Verification items for the finished model (mm, model axes). Round coordinates to 2 decimals unless told otherwise and drop trailing zeros. Write each loop counter-clockwise with the first axis right and the second up, starting at its lowest first coordinate (ties: lowest second). Pieces come first, ordered by that corner, then holes. Notation, with made-up numbers: (-8.75, -32) -> (49.25, -32) arc R25 ccw to (49.25, 6) -> close; hole circle Ø7 at (-40, 44). An arc over 180 degrees is marked (long way). Answer as a JSON object with one key per item and string values. Group by question number.
(1) Sectioned sample at B-B on x = 3.6. Count the separate pieces of the cut face and the enclosed holes in it, and give its area (3 significant figures).
(2) Scan lines: L1, parallel to Z at x = 0.3, y = 90.5; L2, parallel to Z at x = 4.1, y = 73; L3, parallel to Z at x = 4.7, y = 118. Record each from-to range of solid material in increasing order. Write a range as from..to.
(3) Sectioned sample at A-A on y = 152. Record the cut outline in (x, z).
(4) Gauge pin test, flat ends, axial feed: pin 1 Ø4.5 at (y, z) = (116.92, -299.36) entering from +X; pin 2 Ø3 at (x, y) = (2, 155.5) entering from -Z; pin 3 Ø3 at (x, y) = (3, 252.5) entering from +Z; pin 4 Ø1.8 at (x, y) = (1.5, 113.5) entering from +Z. Record the tip position at first contact, or that the pin passes through.
(5) Sectioned sample at C-C on y = 243.5. Record the cut outline in (x, z).
```python
from build123d import *

# Parameters (mm, degrees)
SKETCH3_W           = 420
SKETCH3_H           = 170
BOSS_EXTRUDE2_DEPTH = 6
SKETCH4_W           = 6.1
SKETCH4_H           = 85
SKETCH4_W_2         = 6.2
CUT_EXTRUDE1_DEPTH  = 6
SKETCH5_R           = 2
CUT_EXTRUDE2_DEPTH  = 6
SKETCH6_W           = 6
SKETCH6_H           = 380
BOSS_EXTRUDE3_DEPTH = 30
SKETCH7_W           = 6
SKETCH7_H           = 380
CUT_EXTRUDE3_DEPTH  = 2
SKETCH8_W           = 6
SKETCH8_H           = 116.9
SKETCH8_H_2         = 133.8
BOSS_EXTRUDE4_DEPTH = 28
SKETCH9_W           = 6
SKETCH9_H           = 6.2
BOSS_EXTRUDE5_DEPTH = 113
SKETCH10_W          = 6
SKETCH10_H          = 6.2
BOSS_EXTRUDE6_DEPTH = 113
SKETCH11_W          = 6.2
SKETCH11_H          = 113
CUT_EXTRUDE4_DEPTH  = 113
SKETCH12_W          = 6
SKETCH12_H          = 10
CUT_EXTRUDE6_DEPTH  = 1000
SKETCH13_W          = 20
SKETCH13_H          = 10
SKETCH13_W_2        = 13.9
CUT_EXTRUDE7_DEPTH  = 1000


with BuildPart() as part:
    # Sketch3 → Boss-Extrude2 (new body)
    with BuildSketch(Plane(origin=(0, 0, 0), x_dir=(0, 0, -1), z_dir=(1, 0, 0))):
        with Locations((440.911700258, 161.915861829)):
            Rectangle(SKETCH3_W, SKETCH3_H)
    extrude(amount=BOSS_EXTRUDE2_DEPTH)

    # Sketch4 → Cut-Extrude1 (cut)
    with BuildSketch(Plane(origin=(6, 0, 0), x_dir=(0, 0, -1), z_dir=(1, 0, 0))):
        with Locations((233.961700258, 119.415861829)):
            Rectangle(SKETCH4_W, SKETCH4_H)
        with Locations((647.861700258, 119.415861829)):
            Rectangle(SKETCH4_W, SKETCH4_H)
        with Locations((370.911700258, 204.415861829)):
            Rectangle(SKETCH4_W_2, SKETCH4_H)
        with Locations((510.911700258, 204.415861829)):
            Rectangle(SKETCH4_W_2, SKETCH4_H)
    extrude(amount=-CUT_EXTRUDE1_DEPTH, mode=Mode.SUBTRACT)

    # Sketch5 → Cut-Extrude2 (cut)
    with BuildSketch(Plane(origin=(6, 0, 0), x_dir=(0, 0, -1), z_dir=(1, 0, 0))):
        with Locations((299.361700258, 206.915861829)):
            Circle(SKETCH5_R)
        with Locations((299.361700258, 116.915861829)):
            Circle(SKETCH5_R)
        with Locations((440.911700258, 206.915861829)):
            Circle(SKETCH5_R)
        with Locations((582.461700258, 206.915861829)):
            Circle(SKETCH5_R)
        with Locations((582.461700258, 116.915861829)):
            Circle(SKETCH5_R)
        with Locations((440.911700258, 116.915861829)):
            Circle(SKETCH5_R)
    extrude(amount=-CUT_EXTRUDE2_DEPTH, mode=Mode.SUBTRACT)

    # Sketch6 → Boss-Extrude3 (add)
    with BuildSketch(Plane.XZ.offset(-76.915861829)):
        with Locations((3, -440.911700258)):
            Rectangle(SKETCH6_W, SKETCH6_H)
    extrude(amount=BOSS_EXTRUDE3_DEPTH)

    # Sketch7 → Cut-Extrude3 (cut)
    with BuildSketch(Plane.XZ.offset(-46.915861829)):
        with Locations((3, -440.911700258)):
            Rectangle(SKETCH7_W, SKETCH7_H)
    extrude(amount=-CUT_EXTRUDE3_DEPTH, mode=Mode.SUBTRACT)

    # Sketch8 → Boss-Extrude4 (add)
    with BuildSketch(Plane(origin=(0, 246.915861829, 0), x_dir=(1, 0, 0), z_dir=(0, 1, 0))):
        with Locations((3, 309.361700258)):
            Rectangle(SKETCH8_W, SKETCH8_H)
        with Locations((3, 572.461700258)):
            Rectangle(SKETCH8_W, SKETCH8_H)
        with Locations((3, 440.911700258)):
            Rectangle(SKETCH8_W, SKETCH8_H_2)
    extrude(amount=BOSS_EXTRUDE4_DEPTH)

    # Sketch9 → Boss-Extrude5 (add)
    with BuildSketch(Plane(origin=(0, 161.915861829, 0), x_dir=(1, 0, 0), z_dir=(0, 1, 0))):
        with Locations((3, 370.911700258)):
            Rectangle(SKETCH9_W, SKETCH9_H)
    extrude(amount=BOSS_EXTRUDE5_DEPTH)

    # Sketch10 → Boss-Extrude6 (add)
    with BuildSketch(Plane(origin=(0, 161.915861829, 0), x_dir=(1, 0, 0), z_dir=(0, 1, 0))):
        with Locations((3, 510.911700258)):
            Rectangle(SKETCH10_W, SKETCH10_H)
    extrude(amount=BOSS_EXTRUDE6_DEPTH)

    # Sketch11 → Cut-Extrude4 (cut)
    with BuildSketch(Plane(origin=(6, 0, 0), x_dir=(0, 0, -1), z_dir=(1, 0, 0))):
        with Locations((370.911700258, 105.415861829)):
            Rectangle(SKETCH11_W, SKETCH11_H)
        with Locations((510.911700258, 105.415861829)):
            Rectangle(SKETCH11_W, SKETCH11_H)
    extrude(amount=-CUT_EXTRUDE4_DEPTH, mode=Mode.SUBTRACT)

    # Sketch12 → Cut-Extrude6 (cut)
    with BuildSketch(Plane.XY.offset(-250.911700258)):
        with Locations((3, 269.515338883)):
            Rectangle(SKETCH12_W, SKETCH12_H)
        with Locations((3, 53.915861829)):
            Rectangle(SKETCH12_W, SKETCH12_H)
    extrude(amount=-CUT_EXTRUDE6_DEPTH, mode=Mode.SUBTRACT)


with BuildPart() as body_2:
    # of the pieces the cut leaves, the one that is kept (cut_extrude6_keep)
    add(part.part.solids().sort_by_distance((0, 76.915861829, -237.011700258))[0])

    # Sketch13 → Cut-Extrude7 (cut)
    with BuildSketch(Plane(origin=(6, 0, 0), x_dir=(0, 0, -1), z_dir=(1, 0, 0))):
        with Locations((240.911700258, 241.915861829)):
            Rectangle(SKETCH13_W, SKETCH13_H)
        with Locations((640.911700258, 241.915861829)):
            Rectangle(SKETCH13_W, SKETCH13_H)
        with Locations((243.961700258, 81.915861829)):
            Rectangle(SKETCH13_W_2, SKETCH13_H)
        with Locations((637.861700258, 81.915861829)):
            Rectangle(SKETCH13_W_2, SKETCH13_H)
    extrude(amount=-CUT_EXTRUDE7_DEPTH, mode=Mode.SUBTRACT)


solid = body_2.part
```
Computed values:
{
 "1": {"separate pieces": "1", "enclosed holes": "6", "area": "81,900 mm2"},
 "2": {"L1": "-644.81..-514.01, -507.81..-374.01, -367.81..-237.01", "L2": "-630.91..-514.01, -507.81..-374.01, -367.81..-250.91", "L3": "-644.81..-584.14, -580.78..-514.01, -507.81..-442.59, -439.23..-374.01, -367.81..-301.04, -297.68..-237.01"},
 "3": {"outline": "(0, -644.81) -> (6, -644.81) -> (6, -514.01) -> (0, -514.01) -> close; (0, -507.81) -> (6, -507.81) -> (6, -374.01) -> (0, -374.01) -> close; (0, -367.81) -> (6, -367.81) -> (6, -237.01) -> (0, -237.01) -> close"},
 "4": {"pin 1": "x = 6", "pin 2": "z = -644.81", "pin 3": "z = -250.91", "pin 4": "z = -237.01"},
 "5": {"outline": "(0, -630.91) -> (6, -630.91) -> (6, -250.91) -> (0, -250.91) -> close"}
}
